The listing builds one solid part. Answer for the finished solid, in the listing's coordinates (mm). Give positions to 0.01 mm unless a question says otherwise; leave off trailing zeros. Put each result on its own line as item: value. Start each with the question number.
1) A flat-ended cylindrical pin translates along its axis: pin 1 Ø1 at (x, y) = (-14, 3) entering from +Z. Find the tip coordinate at first contact, or state that the pin passes through.
2) A cutting plane is placed at A-A (y = 3). Give the number of separate pieces and of enclosed holes in the cut face, then the cut area to 3 significant figures.
3) Find the intervals of material crossed by line 1 along Z through (x, y) = (-52.5, 4); line 2 along X through (y, z) = (0.4, 102); line 3 along Z through (x, y) = (-46.5, 2.8), in increasing order. Write a range as from..to.
4) For a pull along X with two mould halves and no side action, classify faces 1 (the flat face through (-91.67, 2.41, -93.35)), 2 (the flat face through (3, 0, 3)), 3 (the flat face through (-48.07, 2.41, 91.67)) as released by +X, released by -X, zero draft, split by the parting line, or undercut.
Autodesk Inventor part; units mm, degrees
ref_plane "YZ Plane" through (0, 0, 0) normal (1, 0, 0) x (0, 1, 0)
ref_plane "XZ Plane" through (0, 0, 0) normal (0, 1, 0) x (-1, 0, 0)
ref_plane "XY Plane" through (0, 0, 0) normal (0, 0, 1) x (1, 0, 0)
sketch "Sketch1" plane through (0, 0, 0) normal (0, 1, 0) x (-1, 0, 0)
  circle A0 centre (0, 0) radius 200
  dimension "d0" = 400
extrude "Extrusion1" add sketch "Sketch1" along normal blind 4.7625
chamfer "Chamfer1" distance 2 angle 12.5 1 edges at (200, 0, 0) measured on face at (94.1877, 1.5875, -176.4332)
sketch "Sketch2" plane through (0, 4.7625, 0) normal (0, 1, 0) x (1, 0, 0)
  line L0 (0, 0) -> (200, 0) construction
  line L1 (0, 0) -> (160, 0) construction
  line L2 (0, 0) -> (100, 0) construction
  line L3 (88.3859, -54.7142) -> (54.7142, -88.3859)
  line L4 (54.7142, -88.3859) -> (53.0355, -86.7072)
  line L5 (53.0355, -86.7072) -> (86.7072, -53.0355)
  line L6 (88.3859, -54.7142) -> (86.7072, -53.0355)
  line L7 (54.7142, -53.0355) -> (53.0355, -54.7142)
  line L8 (53.0355, -54.7142) -> (86.7072, -88.3859)
  line L9 (86.7072, -88.3859) -> (88.3859, -86.7072)
  line L10 (88.3859, -86.7072) -> (54.7142, -53.0355)
  circle A0 centre (0, 0) radius 200
  line L11 (-88.3859, -54.7142) -> (-54.7142, -88.3859)
  line L12 (-54.7142, -88.3859) -> (-53.0355, -86.7072)
  line L13 (-53.0355, -86.7072) -> (-86.7072, -53.0355)
  line L14 (-88.3859, -54.7142) -> (-86.7072, -53.0355)
  line L15 (-54.7142, -53.0355) -> (-53.0355, -54.7142)
  line L16 (-53.0355, -54.7142) -> (-86.7072, -88.3859)
  line L17 (-86.7072, -88.3859) -> (-88.3859, -86.7072)
  line L18 (-88.3859, -86.7072) -> (-54.7142, -53.0355)
  line L19 (88.3859, 54.7142) -> (54.7142, 88.3859)
  line L20 (54.7142, 88.3859) -> (53.0355, 86.7072)
  line L21 (53.0355, 86.7072) -> (86.7072, 53.0355)
  line L22 (88.3859, 54.7142) -> (86.7072, 53.0355)
  line L23 (54.7142, 53.0355) -> (53.0355, 54.7142)
  line L24 (53.0355, 54.7142) -> (86.7072, 88.3859)
  line L25 (86.7072, 88.3859) -> (88.3859, 86.7072)
  line L26 (88.3859, 86.7072) -> (54.7142, 53.0355)
  line L27 (-88.3859, 54.7142) -> (-54.7142, 88.3859)
  line L28 (-54.7142, 88.3859) -> (-53.0355, 86.7072)
  line L29 (-53.0355, 86.7072) -> (-86.7072, 53.0355)
  line L30 (-53.0355, 54.7142) -> (-86.7072, 88.3859)
  line L31 (-88.3859, 86.7072) -> (-54.7142, 53.0355)
  line L32 (-86.7072, 88.3859) -> (-88.3859, 86.7072)
  line L33 (-88.3859, 54.7142) -> (-86.7072, 53.0355)
  line L34 (-54.7142, 53.0355) -> (-53.0355, 54.7142)
  point P0 (69.032, 70.7107)
  point P1 (70.7107, 69.032)
  point P2 (72.3893, 70.7107)
  point P3 (70.7107, 72.3893)
  point P4 (-69.032, 70.7107)
  point P5 (-70.7107, 72.3893)
  point P6 (-72.3893, 70.7107)
  point P7 (-70.7107, 69.032)
  point P8 (-72.3893, -70.7107)
  point P9 (-70.7107, -72.3893)
  point P10 (-69.032, -70.7107)
  point P11 (-70.7107, -69.032)
  point P12 (72.3893, -70.7107)
  point P13 (70.7107, -69.032)
  point P14 (69.032, -70.7107)
  point P15 (70.7107, -72.3893)
  dimension "d16" = 2.374
  dimension "d20" = 47.619
extrude "Extrusion2" cut sketch "Sketch2" against normal blind 10 contours L3 L10 L5 L6 | L10 L9 L8 L3 | L3 L8 L5 L10 | L3 L4 L5 L8 | L5 L8 L7 L10 | L14 L13 L18 L11 | L18 L13 L16 L11 | L11 L16 L17 L18 | L16 L13 L12 L11 | L18 L15 L16 L13 | L22 L21 L26 L19 | L26 L21 L24 L19 | L19 L24 L25 L26 | L24 L21 L20 L19 | L26 L23 L24 L21 | L27 L31 L29 L33 | L31 L32 L30 L27 | L27 L30 L29 L31 | L27 L28 L29 L30 | L29 L30 L34 L31
sketch "Sketch3" plane through (0, 4.7625, 0) normal (0, 1, 0) x (1, 0, 0)
  line L0 (-54.7142, 53.0355) -> (-28.1977, 26.519)
  line L1 (-53.0355, 54.7142) -> (-26.519, 28.1977)
  line L2 (-26.519, 28.1977) -> (-28.1977, 26.519)
  line L3 (-53.0355, 54.7142) -> (-54.7142, 53.0355)
  line L4 (-88.3859, 86.7072) -> (-114.9024, 113.2237)
  line L5 (-86.7072, 88.3859) -> (-113.2237, 114.9024)
  line L6 (-113.2237, 114.9024) -> (-114.9024, 113.2237)
  line L7 (-86.7072, 88.3859) -> (-88.3859, 86.7072)
  line L8 (-54.7142, 88.3859) -> (-53.0355, 86.7072)
  line L9 (-53.0355, 86.7072) -> (-26.519, 113.2237)
  line L10 (-54.7142, 88.3859) -> (-28.1977, 114.9024)
  line L11 (-28.1977, 114.9024) -> (-26.519, 113.2237)
  line L12 (-88.3859, 54.7142) -> (-86.7072, 53.0355)
  line L13 (-86.7072, 53.0355) -> (-113.2237, 26.519)
  line L14 (-88.3859, 54.7142) -> (-114.9024, 28.1977)
  line L15 (-114.9024, 28.1977) -> (-113.2237, 26.519)
  circle A0 centre (0, 0) radius 200
  line L16 (-54.7142, -53.0355) -> (-28.1977, -26.519)
  line L17 (-53.0355, -54.7142) -> (-26.519, -28.1977)
  line L18 (-26.519, -28.1977) -> (-28.1977, -26.519)
  line L19 (-53.0355, -54.7142) -> (-54.7142, -53.0355)
  line L20 (-86.7072, -88.3859) -> (-113.2237, -114.9024)
  line L21 (-86.7072, -88.3859) -> (-88.3859, -86.7072)
  line L22 (-88.3859, -86.7072) -> (-114.9024, -113.2237)
  line L23 (-113.2237, -114.9024) -> (-114.9024, -113.2237)
  line L24 (-54.7142, -88.3859) -> (-53.0355, -86.7072)
  line L25 (-53.0355, -86.7072) -> (-26.519, -113.2237)
  line L26 (-54.7142, -88.3859) -> (-28.1977, -114.9024)
  line L27 (-28.1977, -114.9024) -> (-26.519, -113.2237)
  line L28 (-114.9024, -28.1977) -> (-113.2237, -26.519)
  line L29 (-88.3859, -54.7142) -> (-114.9024, -28.1977)
  line L30 (-86.7072, -53.0355) -> (-113.2237, -26.519)
  line L31 (-88.3859, -54.7142) -> (-86.7072, -53.0355)
  line L32 (54.7142, 53.0355) -> (28.1977, 26.519)
  line L33 (53.0355, 54.7142) -> (26.519, 28.1977)
  line L34 (26.519, 28.1977) -> (28.1977, 26.519)
  line L35 (53.0355, 54.7142) -> (54.7142, 53.0355)
  line L36 (86.7072, 88.3859) -> (113.2237, 114.9024)
  line L37 (86.7072, 88.3859) -> (88.3859, 86.7072)
  line L38 (88.3859, 86.7072) -> (114.9024, 113.2237)
  line L39 (113.2237, 114.9024) -> (114.9024, 113.2237)
  line L40 (54.7142, 88.3859) -> (53.0355, 86.7072)
  line L41 (53.0355, 86.7072) -> (26.519, 113.2237)
  line L42 (54.7142, 88.3859) -> (28.1977, 114.9024)
  line L43 (28.1977, 114.9024) -> (26.519, 113.2237)
  line L44 (114.9024, 28.1977) -> (113.2237, 26.519)
  line L45 (88.3859, 54.7142) -> (114.9024, 28.1977)
  line L46 (86.7072, 53.0355) -> (113.2237, 26.519)
  line L47 (88.3859, 54.7142) -> (86.7072, 53.0355)
  line L48 (54.7142, -88.3859) -> (28.1977, -114.9024)
  line L49 (53.0355, -86.7072) -> (26.519, -113.2237)
  line L50 (54.7142, -88.3859) -> (53.0355, -86.7072)
  line L51 (28.1977, -114.9024) -> (26.519, -113.2237)
  line L52 (53.0355, -54.7142) -> (54.7142, -53.0355)
  line L53 (53.0355, -54.7142) -> (26.519, -28.1977)
  line L54 (54.7142, -53.0355) -> (28.1977, -26.519)
  line L55 (26.519, -28.1977) -> (28.1977, -26.519)
  line L56 (88.3859, -54.7142) -> (86.7072, -53.0355)
  line L57 (88.3859, -54.7142) -> (114.9024, -28.1977)
  line L58 (86.7072, -53.0355) -> (113.2237, -26.519)
  line L59 (114.9024, -28.1977) -> (113.2237, -26.519)
  line L60 (88.3859, -86.7072) -> (114.9024, -113.2237)
  line L61 (86.7072, -88.3859) -> (113.2237, -114.9024)
  line L62 (113.2237, -114.9024) -> (114.9024, -113.2237)
  line L63 (86.7072, -88.3859) -> (88.3859, -86.7072)
extrude "Extrusion3" cut sketch "Sketch3" against normal blind 10 contours L3 L1 L2 L0 | L4 L6 L5 L7 | L10 L11 L9 L8 | L12 L13 L15 L14 | L16 L18 L17 L19 | L20 L23 L22 L21 | L24 L25 L27 L26 | L28 L30 L31 L29 | L32 L34 L33 L35 | L36 L39 L38 L37 | L40 L41 L43 L42 | L44 L46 L47 L45 | L48 L51 L49 L50 | L53 L55 L54 L52 | L56 L58 L59 L57 | L60 L62 L61 L63
properties part number "Sustainable Chair_V2 - Seat" material "Foam Board - V3"
Reply:
1. pin 1: stops at z = 199.54
2. separate pieces: 1
2. enclosed holes: 4
2. area: 123,000 mm2
3. line 1: z = -192.99..-90.6, -87.24..-54.18, -50.82..50.82, 54.18..87.24, 90.6..192.99
3. line 2: x = -171.62..-103.68, -100.32..-41.1, -37.74..37.74, 41.1..100.32, 103.68..171.62
3. line 3: z = -194.52..-96.6, -93.24..-48.18, -44.82..44.82, 48.18..93.24, 96.6..194.52
4. face 1: undercut
4. face 2: zero draft
4. face 3: undercut
